Source: CAD feature listing. Evaluate the final solid. Frame: model axes, mm. A direction names the side the tool comes from. Round coordinates to 2 decimals unless told otherwise and drop trailing zeros. Order: outer loops, then holes, each group sorted by start corner. A loop starts at its lowest first (then second) coordinate and runs counter-clockwise, first axis right, second up. Notation, with made-up numbers: (25, 64) - (73, 64) arc R29 ccw to (73, 89) - close; hole circle Ø8 at (21.5, 77). An arc over 180 degrees is marked (long way). Return JSON: item names as keys, results as strings. Group by question number.
1) Section C-C, the plane x = -5.5. Return loops of the section in (y, z), plus the area to 3 significant figures.
2) Mould query, pull axis X, two halves, no side actions, for faces 1 (the cylindrical face through (-8.66, 0.87, -7.51)), 2 (the cylindrical face through (-6.89, -2.11, 8.02)), 3 (the flat face through (25, 1, 0)), 4 (the flat face through (0, -1, 35)). Classes: pulls with the +X half, pulls with the -X half, needs draft (parallel to the pull), parting line crosses it, or undercut.
3) Access query for faces 5 (the cylindrical face through (24, 2, -23)), 6 (the flat face through (-25, 1, 0)), 7 (the flat face through (0, -2.9, 0)). Directions: +Z, -Z, +X, -X, +Y, -Y. A direction counts if a zero-diameter tool reaches every point of the face in a straight line with its end or side. Return the directions, or none.
4) Section A-A, the plane x = 11. Return loops of the section in (y, z), plus the area to 3 significant figures.
5) Contact query for flat-ended pins moving along their axis: P1, Ø6, axis at x = -5.5, z = -9.53, coming from the +Y side; P2, Ø1.5, axis at x = -1.5, y = 1, coming from the +Z side; P3, Ø1.5, axis at x = 9, y = 1.5, coming from the -Z side. Output: stop coordinate, or through.
6) Section D-D, the plane z = 24. Return loops of the section in (x, y).
7) Ray query, line 1 (Z direction, x = -8, y = 1.55); line 2 (Z direction, x = 11, y = -2); line 3 (X direction, y = 0.8, z = 0). Return the intervals inside material, ascending. Write a range as from..to.
8) Section B-B, the plane z = 0. Return loops of the section in (x, y).
Autodesk Inventor part; units mm, degrees
ref_plane "YZ Plane" through (0, 0, 0) normal (1, 0, 0) x (0, 1, 0)
ref_plane "XZ Plane" through (0, 0, 0) normal (0, 1, 0) x (-1, 0, 0)
ref_plane "XY Plane" through (0, 0, 0) normal (0, 0, 1) x (1, 0, 0)
sketch "Sketch1" plane through (0, 0, 0) normal (0, 1, 0) x (-1, 0, 0)
  line L0 (-35, 35) -> (35, 35)
  line L1 (35, 35) -> (35, -35)
  line L2 (35, -35) -> (-35, -35)
  line L3 (-35, -35) -> (-35, 35)
  line L4 (-35, 35) -> (35, -35) construction
  line L5 (35, 35) -> (-35, -35) construction
  line L6 (-25, 25) -> (25, 25)
  line L7 (25, 25) -> (25, -25)
  line L8 (25, -25) -> (-25, -25)
  line L9 (-25, -25) -> (-25, 25)
  line L10 (-25, 25) -> (25, -25) construction
  line L11 (25, 25) -> (-25, -25) construction
  circle A0 centre (0, 0) radius 15 construction
  circle A1 centre (0, 0) radius 11 construction
  point P0 (15, 0)
  dimension "d4" = 30
  dimension "d0" = 70
  dimension "d1" = 70
  dimension "d2" = 50
  dimension "d3" = 50
  dimension "d5" = 22
extrude "Extrusion1" add sketch "Sketch1" along normal blind 3 contours L6 L7 L8 L9
extrude "Extrusion2" add sketch "Sketch1" against normal blind 3 contours L0 L1 L2 L3 | L6 L7 L8 L9
sketch "Sketch2" plane through (0, 3, 0) normal (0, 1, 0) x (1, 0, 0)
  circle A0 centre (0, 0) radius 11 construction
  circle A1 centre (0, 0) radius 15 construction
  point P0 (11, 0)
hole "Hole1" at (11, 3, 0) direction (0, -1, 0) diameter 4.1 end through all counterbore diameter 7.5 counterbore depth 4.2
pattern_circular "Circular Pattern1" count 3 over 360 about axis through (0, 3, 0) along (0, -1, 0) of "Hole1"
fillet "Fillet1" radius 5 8 edges at (35, -1.5, 35) (-35, -1.5, 35) (-35, -1.5, -35) (35, -1.5, -35) (25, 1.5, -25) (25, 1.5, 25) (-25, 1.5, 25) (-25, 1.5, -25)
sketch "Sketch3" plane through (0, -3, 0) normal (0, -1, 0) x (1, 0, 0)
  circle A0 centre (0, 0) radius 1
  dimension "d21" = 2
extrude "Extrusion3" cut sketch "Sketch3" against normal blind 0.1
properties part number "support_plateau_v3"
Geometry check:
{
 "1": {"outline": "(-3, -35) - (0, -35) - (0, -25) - (3, -25) - (3, -13.28) - (-1.2, -13.28) - (-1.2, -11.58) - (-3, -11.58) - close; (-3, -7.48) - (-1.2, -7.48) - (-1.2, -5.78) - (3, -5.78) - (3, 5.78) - (-1.2, 5.78) - (-1.2, 7.48) - (-3, 7.48) - close; (-3, 11.58) - (-1.2, 11.58) - (-1.2, 13.28) - (3, 13.28) - (3, 25) - (0, 25) - (0, 35) - (-3, 35) - close", "area": "282 mm2"},
 "2": {"face 1": "undercut", "face 2": "undercut", "face 3": "pulls with the +X half", "face 4": "needs draft"},
 "3": {"face 5": "-Z, +X, +Y", "face 6": "+Z, -Z, -X, +Y", "face 7": "-Y"},
 "4": {"outline": "(-3, -35) - (0, -35) - (0, -25) - (3, -25) - (3, -3.75) - (-1.2, -3.75) - (-1.2, -2.05) - (-3, -2.05) - close; (-3, 2.05) - (-1.2, 2.05) - (-1.2, 3.75) - (3, 3.75) - (3, 25) - (0, 25) - (0, 35) - (-3, 35) - close", "area": "321 mm2"},
 "5": {"P1": "y = -1.2", "P2": "z = 25", "P3": "z = -25"},
 "6": {"outline": "(-35, -3) - (35, -3) - (35, 0) - (23, 0) - (23, 3) - (-23, 3) - (-23, 0) - (-35, 0) - close"},
 "7": {"line 1": "-25..-12.32, -6.73..6.73, 12.32..25", "line 2": "-35..-2.05, 2.05..35", "line 3": "-25..7.25, 14.75..25"},
 "8": {"outline": "(-35, -3) - (-1, -3) - (-1, -2.9) - (1, -2.9) - (1, -3) - (8.95, -3) - (8.95, -1.2) - (7.25, -1.2) - (7.25, 3) - (-25, 3) - (-25, 0) - (-35, 0) - close; (13.05, -3) - (35, -3) - (35, 0) - (25, 0) - (25, 3) - (14.75, 3) - (14.75, -1.2) - (13.05, -1.2) - close"}
}
